Verification items for this drawing (mm, ordinates from the low corner). Round coordinates to 2 decimals unless told otherwise and drop trailing zeros. Loops run counter-clockwise (first coordinate to the right, second up) from the corner with the lowest first, then second, coordinate; pieces in that order, holes last. Notation, with made-up numbers: (9, 87) -> (36, 87) arc R18 cw to (36, 108) -> close; hole circle Ø10 at (41.25, 66). An arc over 180 degrees is marked (long way). One line per item, written item: value. Start each with the question number.
1. Cross-section at C-C on x = 38.1. Record the cut outline in (y, z).
2. Go/stop test with a flat-tipped pin: pin 1 (8 mm diameter, centred on x = 33, z = 35, fed in from +Y). Record where the tip stops, or that it passes through.
3. Cross-section at A-A on y = 0.85. Record the cut outline in (x, z) (3 decimals).
4. Cross-section at B-B on z = 6. Record the cut outline in (x, y).
5. Material ranges on L1, parallel to X at y = 0.8, z = 38; L2, parallel to X at y = 3.8, z = 32.5, recorded low to high.
6. Cross-section at D-D on z = 38.1. Record the cut outline in (x, y), then the cut area to 3 significant figures.
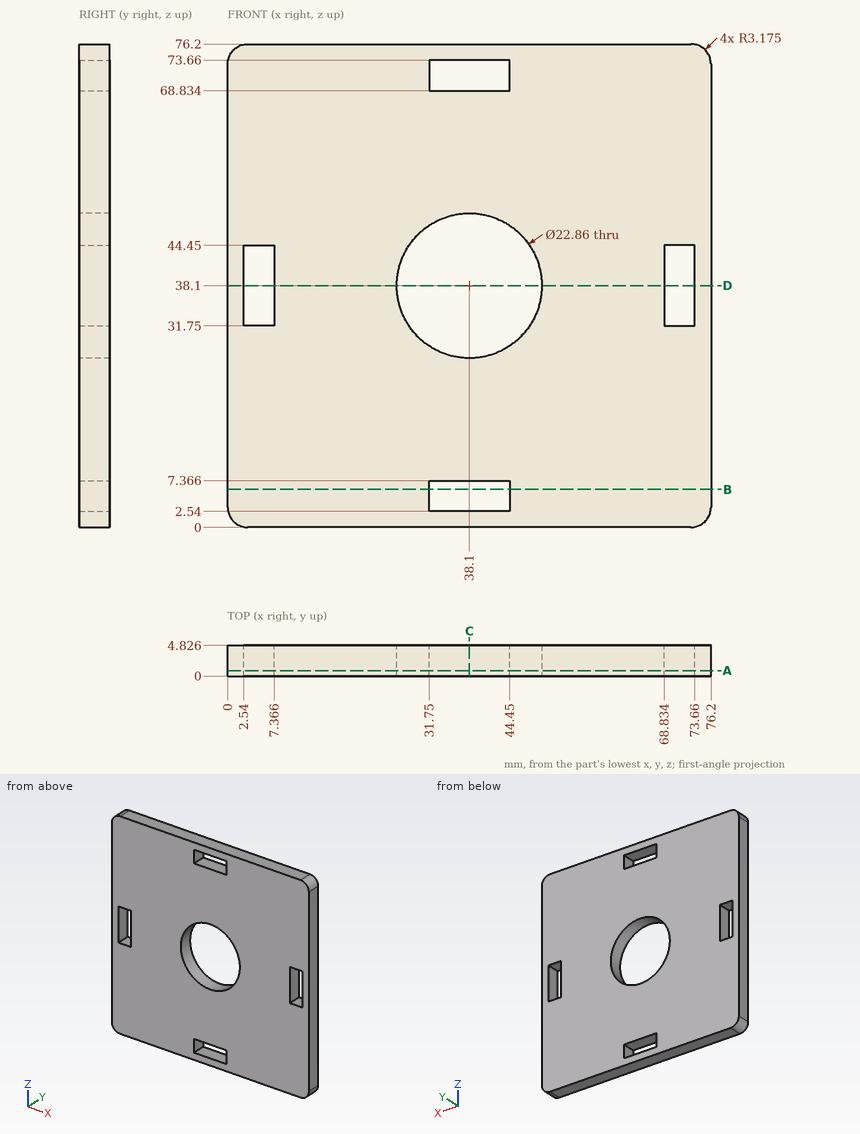
Taken from the geometry:
1. outline: (0, 0) -> (4.83, 0) -> (4.83, 2.54) -> (0, 2.54) -> close; (0, 7.37) -> (4.83, 7.37) -> (4.83, 26.67) -> (0, 26.67) -> close; (0, 49.53) -> (4.83, 49.53) -> (4.83, 68.83) -> (0, 68.83) -> close; (0, 73.66) -> (4.83, 73.66) -> (4.83, 76.2) -> (0, 76.2) -> close
2. pin 1: passes through
3. outline: (0, 3.175) arc R3.175 ccw to (3.175, 0) -> (73.025, 0) arc R3.175 ccw to (76.2, 3.175) -> (76.2, 73.025) arc R3.175 ccw to (73.025, 76.2) -> (3.175, 76.2) arc R3.175 ccw to (0, 73.025) -> close; hole (2.54, 31.75) -> (7.366, 31.75) -> (7.366, 44.45) -> (2.54, 44.45) -> close; hole circle Ø22.86 at (38.1, 38.1); hole (31.75, 2.54) -> (44.45, 2.54) -> (44.45, 7.366) -> (31.75, 7.366) -> close; hole (31.75, 68.834) -> (44.45, 68.834) -> (44.45, 73.66) -> (31.75, 73.66) -> close; hole (68.834, 31.75) -> (73.66, 31.75) -> (73.66, 44.45) -> (68.834, 44.45) -> close
4. outline: (0, 0) -> (31.75, 0) -> (31.75, 4.83) -> (0, 4.83) -> close; (44.45, 0) -> (76.2, 0) -> (76.2, 4.83) -> (44.45, 4.83) -> close
5. L1: x = 0 to 2.54, 7.37 to 26.67, 49.53 to 68.83, 73.66 to 76.2
5. L2: x = 0 to 2.54, 7.37 to 28.14, 48.06 to 68.83, 73.66 to 76.2
6. outline: (0, 0) -> (2.54, 0) -> (2.54, 4.83) -> (0, 4.83) -> close; (7.37, 0) -> (26.67, 0) -> (26.67, 4.83) -> (7.37, 4.83) -> close; (49.53, 0) -> (68.83, 0) -> (68.83, 4.83) -> (49.53, 4.83) -> close; (73.66, 0) -> (76.2, 0) -> (76.2, 4.83) -> (73.66, 4.83) -> close
6. area: 211 mm2
